Geometry check sheet. Reference: the model listing, model coordinates, mm. Face numbers are marked on the shaded views. A direction names the side the tool comes from. Coordinates: 2 decimals unless noted, no trailing zeros. Write each loop counter-clockwise with the first axis right and the second up, starting at its lowest first coordinate (ties: lowest second). Pieces come first, ordered by that corner, then holes. Notation, with made-up numbers: (-16.75, 48) -> (41.25, 48) arc R24 ccw to (41.25, 82) -> close; hole circle Ø10 at (32.25, 61). An arc over 180 degrees is marked (long way). Answer in a Markdown table with one row per item. Add a question column.
Q1. Thickness scan on line 1 (Y direction, x = 10, z = 1.5); line 2 (Z direction, x = -6.25, y = 4.25); line 3 (X direction, y = 9.75, z = 1.75). Record the ranges inside material, lowest first.
Q2. Section check B-B, the plane x = 10. Record the boundary of the cut face in (y, z), and give its area (3 significant figures).
Q3. Section check D-D, the plane z = 1.25. Record the boundary of the cut face in (x, y).
Q4. Section check A-A, the plane y = 7.5. Record the boundary of the cut face in (x, z), and give its area (3 significant figures).
Q5. Section check C-C, the plane z = 3.75. Record the boundary of the cut face in (x, y), and give its area (3 significant figures).
Q6. Tool access check on the marked faces 1, 2, 3 and 4. Record the directions out of +Z, -Z, +X, -X, +Y, -Y that give a thin tool (end or side, any length) a straight path to the whole face; none if there is none.
Q7. Gauge pin test, flat ends, axial feed: P1, Ø4, axis at x = -11.5, z = 5, coming from the -Y side; P2, Ø4.5, axis at x = 8, y = 4, coming from the +Z side. Record the tip position at first contact, or that the pin passes through.
Q8. Release check for a two-part mould opening along Y. For the marked faces 5, 6 and 7 record: pulls with the +Y half, pulls with the -Y half, needs draft (parallel to the pull), parting line crosses it, or undercut.
```python
from build123d import *

# Parameters (mm, degrees)
F1_DEPTH = 15
F2_R     = 1.6
F3_DEPTH = 2.901
F4_R     = 2


with BuildPart() as f1:
    # F0 (on Front) → F1 (new body)
    with BuildSketch(Plane.XZ):
        with BuildLine():
            Line((-15, 2.9), (-15, 0))
            Line((-15, 0), (-2.9, 0))
            Line((-2.9, 0), (-2.9, 2.9))
            ThreePointArc((-2.9, 2.9), (0, 5.8), (2.9, 2.9))
            Line((2.9, 2.9), (2.9, 0))
            Line((2.9, 0), (15, 0))
            Line((15, 0), (15, 2.9))
            Line((15, 2.9), (4.25, 2.9))
            ThreePointArc((4.25, 2.9), (0, 7.15), (-4.25, 2.9))
            Line((-4.25, 2.9), (-15, 2.9))
        make_face()
    extrude(amount=-F1_DEPTH)

    # F2 (on face) → F3 (cut, through all)
    with BuildSketch(Plane.XY.offset(2.9)):
        with Locations((-10, 7.5)):
            Circle(F2_R)
        with Locations((10, 7.5)):
            Circle(F2_R)
    extrude(amount=-F3_DEPTH, mode=Mode.SUBTRACT)

    # F4
    f4_edges = [f1.edges().sort_by_distance(p)[0] for p in [
        (-15, 7.5, 2.9),
        (15, 7.5, 2.9),
    ]]
    fillet(f4_edges, radius=F4_R)


solid = f1.part
```
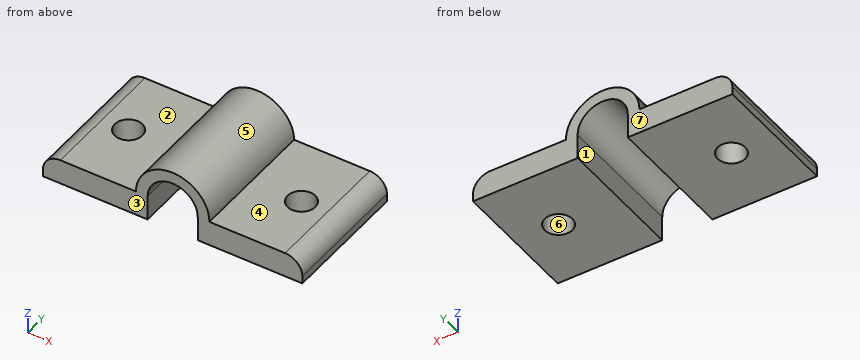
Calculated:
| question | item | result |
|---|---|---|
| 1 | line 1 | y = 0 to 5.9, 9.1 to 15 |
| 1 | line 2 | z = 0 to 2.9 |
| 1 | line 3 | x = -14.81 to -2.9, 2.9 to 14.81 |
| 2 | outline | (0, 0) -> (5.9, 0) -> (5.9, 2.9) -> (0, 2.9) -> close; (9.1, 0) -> (15, 0) -> (15, 2.9) -> (9.1, 2.9) -> close |
| 2 | area | 34.2 mm² |
| 3 | outline | (-14.97, 0) -> (-2.9, 0) -> (-2.9, 15) -> (-14.97, 15) -> close; (2.9, 0) -> (14.97, 0) -> (14.97, 15) -> (2.9, 15) -> close; hole circle Ø3.2 at (-10, 7.5); hole circle Ø3.2 at (10, 7.5) |
| 4 | outline | (-15, 0) -> (-11.6, 0) -> (-11.6, 2.9) -> (-13, 2.9) arc R2 ccw to (-15, 0.9) -> close; (-8.4, 0) -> (-2.9, 0) -> (-2.9, 2.9) arc R2.9 cw to (2.9, 2.9) -> (2.9, 0) -> (8.4, 0) -> (8.4, 2.9) -> (4.25, 2.9) arc R4.25 ccw to (-4.25, 2.9) -> (-8.4, 2.9) -> close; (11.6, 0) -> (15, 0) -> (15, 0.9) arc R2 ccw to (13, 2.9) -> (11.6, 2.9) -> close |
| 4 | area | 65.1 mm² |
| 5 | outline | (-4.16, 0) -> (-2.77, 0) -> (-2.77, 15) -> (-4.16, 15) -> close; (2.77, 0) -> (4.16, 0) -> (4.16, 15) -> (2.77, 15) -> close |
| 5 | area | 41.7 mm² |
| 6 | face 1 | -Z, +Y, -Y |
| 6 | face 2 | +Z, -X, +Y, -Y |
| 6 | face 3 | +Z, -Z, +X, -X, -Y |
| 6 | face 4 | +Z, +X, +Y, -Y |
| 7 | P1 | passes through |
| 7 | P2 | stops at z = 2.9 |
| 8 | face 5 | needs draft |
| 8 | face 6 | undercut |
| 8 | face 7 | pulls with the +Y half |
